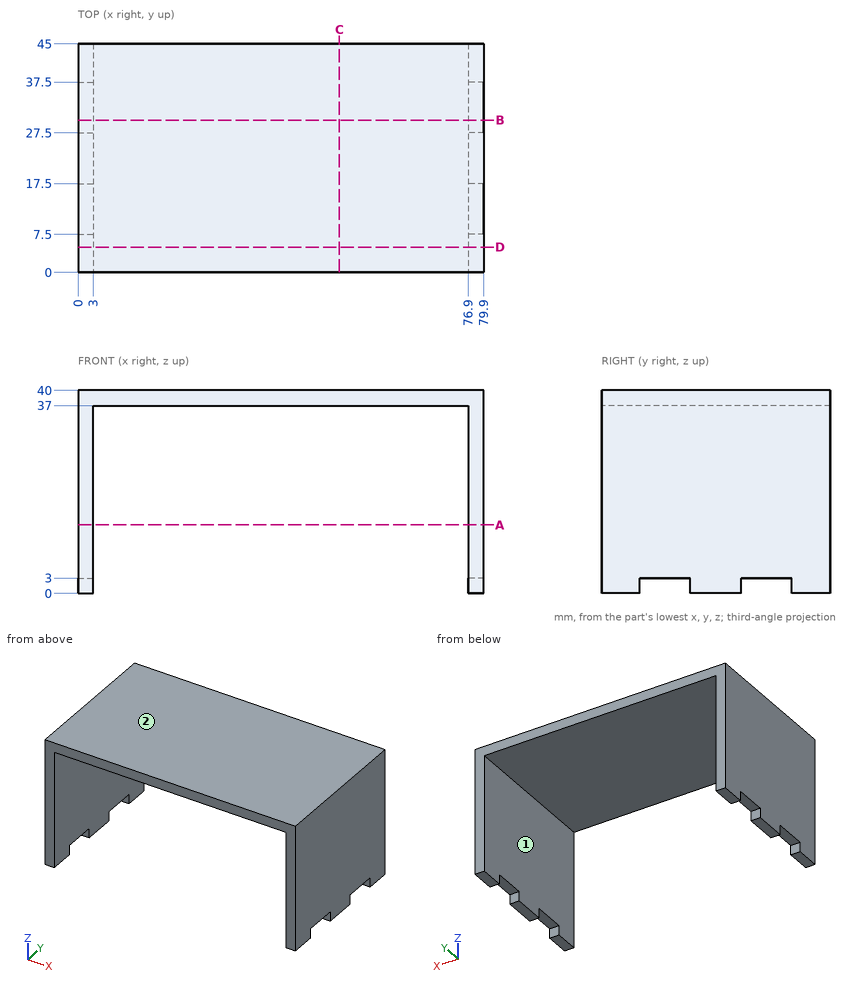
Here's the drawing with two shaded views (mm, measured from the low corner). I have some questions. A direction names the side the tool comes from. Give positions to 0.01 mm unless a question says otherwise; leave off trailing zeros. Write each loop counter-clockwise with the first axis right and the second up, starting at its lowest first coordinate (ties: lowest second). Pieces come first, ordered by that corner, then holes. Notation, with made-up numbers: (-28, -26.75) -> (26, -26.75) arc R28 ccw to (26, 5.25) -> close; hole circle Ø5 at (40, 24.25). An arc over 180 degrees is marked (long way). One line per item, written item: value.
Q1. Imagine slicing it at D-D on y = 5. Please give me the cut outline in (x, z).
Results found:
outline: (0, 0) -> (3, 0) -> (3, 37) -> (76.9, 37) -> (76.9, 0) -> (79.9, 0) -> (79.9, 40) -> (0, 40) -> close
Q2. Imagine slicing it at A-A on z = 13.5. Please give me the cut outline in (x, y).
Results found:
outline: (0, 0) -> (3, 0) -> (3, 45) -> (0, 45) -> close; (76.9, 0) -> (79.9, 0) -> (79.9, 45) -> (76.9, 45) -> close
Q3. For P1, Ø0.9, axis at x = 2, y = 11, coming from the -Z side; P2, Ø13.5, axis at x = 52.5, y = 14.5, coming from the -Z side, each with a flat end and sliding along its axis, tell me the tip position at first contact or that it passes through.
Results found:
P1: stops at z = 3
P2: stops at z = 37
Q4. Please list where these lines run through material, in increasing order: line 1 (X direction, y = 33.5, z = 8); line 2 (Z direction, x = 38, y = 17.5). Write a range as [from, to].
Results found:
line 1: x = [0, 3], [76.9, 79.9]
line 2: z = [37, 40]
Q5. Which directions (+Z, -Z, +X, -X, +Y, -Y) give clear straight access to the entire face, cutting with the end or side of a thin tool? Please do the marked faces 1 and 2.
Results found:
face 1: -Z, +Y, -Y
face 2: +Z, +X, -X, +Y, -Y
Q6. Imagine slicing it at B-B on y = 30. Please give me the cut outline in (x, z).
Results found:
outline: (0, 3) -> (3, 3) -> (3, 37) -> (76.9, 37) -> (76.9, 3) -> (79.9, 3) -> (79.9, 40) -> (0, 40) -> close
Q7. Imagine slicing it at C-C on x = 51.5. Please give me the cut outline in (y, z).
Results found:
outline: (0, 37) -> (45, 37) -> (45, 40) -> (0, 40) -> close
